The figure shows three views and two pictorial views of one solid part (mm, origin at its lowest corner). Answer the questions. Coordinates: 2 decimals unless noted, no trailing zeros. Order: outer loops, then holes, each group sorted by start corner. A loop starts at its lowest first (then second) coordinate and runs counter-clockwise, first axis right, second up. Notation, with made-up numbers: (-8, 35) -> (42, 35) arc R15 ccw to (42, 57) -> close; hole circle Ø2 at (26.5, 53). An arc over 180 degrees is marked (long way). Use one line per item in the form item = value.
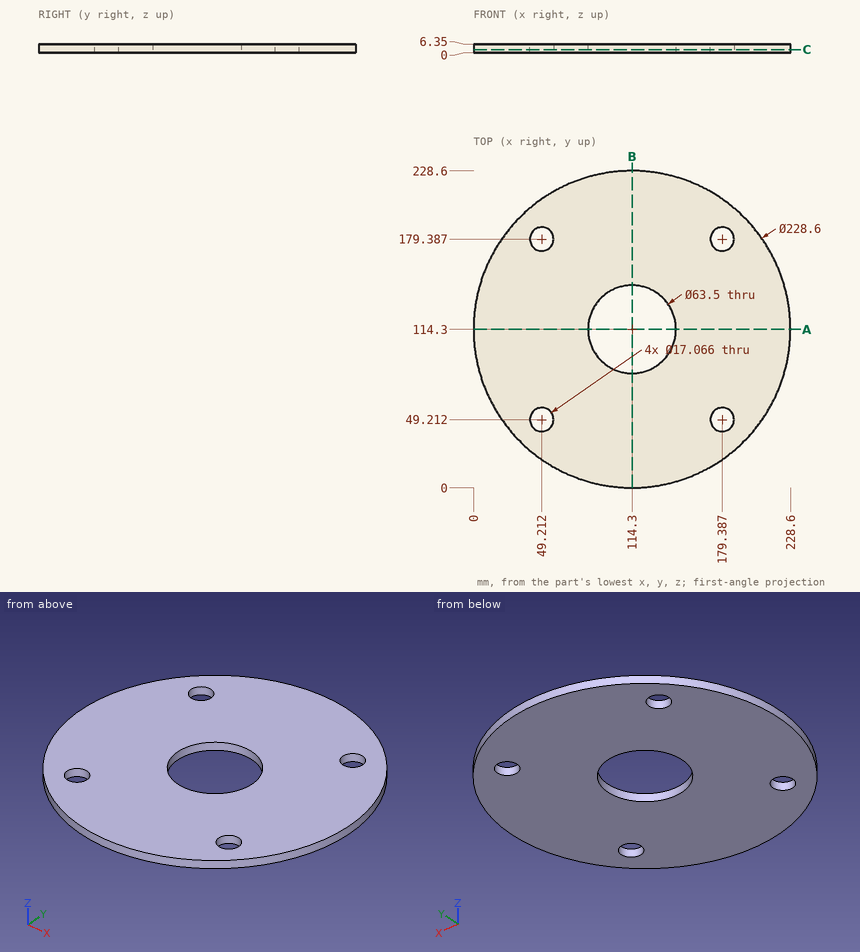
(1) Straight lines are drawn through the part: line 1 along Y through (x, z) = (114.3, 2); line 2 along Y through (x, z) = (46, 0.75); line 3 along X through (y, z) = (95, 3). For each, find the intervals that lie inside material, in ascending order.
Data:
line_1 = 0 to 82.55, 146.05 to 228.6
line_2 = 22.65 to 41.31, 57.12 to 171.48, 187.29 to 205.95
line_3 = 1.64 to 89.09, 139.51 to 226.96
(2) Each of these flat-tipped pins is pushed along its axis until it touches: P1, Ø1.5, axis at y = 82, z = 4.5, coming from the +X side; P2, Ø3, axis at x = 71.5, z = 4, coming from the +Y side; P3, Ø1, axis at y = 101.5, z = 1.5, coming from the +X side. Where does it stop, or does it pass through?
Data:
P1 = 224.16
P2 = 220.88
P3 = 227.94
(3) Section C-C on z = 2.25 is taken. Count the separate pieces of the cut face and the enclosed holes in it, plus the area to 3 significant figures.
Data:
separate_pieces = 1
enclosed_holes = 5
area = 37,000 mm²
(4) Section A-A on y = 114.3 is taken. Write down the section's boundary in (x, z).
Data:
outline = (0, 0) -> (82.55, 0) -> (82.55, 6.35) -> (0, 6.35) -> close; (146.05, 0) -> (228.6, 0) -> (228.6, 6.35) -> (146.05, 6.35) -> close
